```python
from build123d import *

# Parameters (mm, degrees)
F0_W          = 143.1075930595
F0_H          = 104.4075153768
F1_DEPTH      = 12.7
F3_DEPTH      = 25.4
F3_DEPTH_BACK = 25.4
F4_DEPTH      = 25.4
F6_DEPTH      = 25.4


with BuildPart() as f1:
    # F0 (on Top) → F1 (new body)
    with BuildSketch(Plane.XY):
        with Locations((2.4059638381, -20.6538233906)):
            Rectangle(F0_W, F0_H)
    extrude(amount=F1_DEPTH)

    # F2 (on face) → F3 (join, two sides)
    with BuildSketch(Plane.XY.offset(12.7)) as f3_sk:
        with BuildLine():
            Line((15.3577672787, 31.5499342978), (-2.9768298588, 31.5499342978))
            ThreePointArc((-2.9768298588, 31.5499342978), (-24.3292867036, -22.491323871), (4.6469989905, -72.857581079))
            Line((4.6469989905, -72.857581079), (32.5235698655, -72.857581079))
            ThreePointArc((32.5235698655, -72.857581079), (-12.9702679448, -26.7224080826), (15.3577672787, 31.5499342978))
        make_face()
        with BuildLine():
            ThreePointArc((4.6469989905, -72.857581079), (73.6316913936, -76.7914525658), (109.3100037632, -17.6186449826))
            ThreePointArc((109.3100037632, -17.6186449826), (69.2394439219, 43.6714076224), (-2.9768298588, 31.5499342978))
            Line((-2.9768298588, 31.5499342978), (15.3577672787, 31.5499342978))
            ThreePointArc((15.3577672787, 31.5499342978), (42.4015261233, 38.4965408489), (69.4452849679, 31.5499342978))
            Line((69.4452849679, 31.5499342978), (73.9597603679, 31.5499342978))
            Line((73.9597603679, 31.5499342978), (73.9597603679, 28.7816991138))
            ThreePointArc((73.9597603679, 28.7816991138), (91.9989568029, 8.6303350143), (98.5167119547, -17.6186449826))
            ThreePointArc((98.5167119547, -17.6186449826), (91.9989568029, -43.8676249794), (73.9597603679, -64.0189890789))
            Line((73.9597603679, -64.0189890789), (73.9597603679, -72.857581079))
            Line((73.9597603679, -72.857581079), (52.279482381, -72.857581079))
            ThreePointArc((52.279482381, -72.857581079), (42.4015261233, -73.733830814), (32.5235698655, -72.857581079))
            Line((32.5235698655, -72.857581079), (4.6469989905, -72.857581079))
        make_face()
    extrude(amount=F3_DEPTH)
    extrude(f3_sk.sketch, amount=-F3_DEPTH_BACK)

    # F4 (cut): a face of the model
    f4_faces = [f1.faces().sort_by_distance(p)[0] for p in [
        (34.4480932251, -19.6254541978, 12.7),
    ]]
    extrude(f4_faces, amount=-F4_DEPTH, mode=Mode.SUBTRACT)

    # F5 (on Front) → F6 (join)
    with BuildSketch(Plane.XZ):
        Polygon((-24.4303904474, 12.8110842779), (-24.5704315603, 25.2280384302), (-42.8279539842, 12.8110842779), align=None)
    extrude(amount=F6_DEPTH)


solid = f1.part
```
Check sheet for the modelled part. Datum: model origin and axes. Units: mm. A direction names the side the tool comes from. Give positions to 0.01 mm unless a question says otherwise; leave off trailing zeros. Write each loop counter-clockwise with the first axis right and the second up, starting at its lowest first coordinate (ties: lowest second). Pieces come first, ordered by that corner, then holes.
Item 1: Cross-section at B-B (y = 3.5). Enter the section's corners in (x, z).
Item 2: Scan lines: L1, parallel to X at y = -24, z = 23.5 (3 decimals); L2, parallel to Z at x = -57, y = -62; L3, parallel to X at y = 33.5, z = 32. Record each from-to range of solid material in increasing order.
Item 3: Cross-section at A-A (z = 20.5). Enter the section's corners in (x, y).
Item 4: Cross-section at C-C (x = 91). Enter the section's corners in (y, z), and give its area (3 significant figures).
Item 5: Gauge pin test, flat ends, axial feed: pin 1 (2 mm diameter, centred on y = 30, z = 27, fed in from -X); pin 2 (14 mm diameter, centred on x = -31.5, z = 3.5, fed in from +Y); pin 3 (10 mm diameter, centred on x = -31, z = 8, fed in from -Y); pin 4 (5 mm diameter, centred on x = -25.5, y = -17, fed in from +Z). Record the tip position at first contact, or that the pin passes through.
Item 6: Cross-section at D-D (z = 7). Enter the section's corners in (x, y), and give its area (3 significant figures).
Item 7: Access from +Z, -Z, +X, -X, +Y, -Y to the whole of each face (thin tool, end or side, straight path). Record for faces 1 (the face through (-30, -25.4, 16)), 2 (the face through (-37, 31.55, 6)), 3 (the face through (-33, -72.858, 6)), 4 (the face through (-30, 0, 16)), 5 (the face through (7, -62, 38.1)).
Report:
1. outline: (-69.15, 0) - (-21.09, 0) - (-21.09, -12.7) - (-9.59, -12.7) - (-9.59, 38.1) - (-21.09, 38.1) - (-21.09, 12.7) - (-69.15, 12.7) - close; (94.39, -12.7) - (105.89, -12.7) - (105.89, 38.1) - (94.39, 38.1) - close
2. L1: x = -27.111 to -24.551, -24.202 to -13.35, 98.153 to 109.005
2. L2: z = 0 to 12.7
2. L3: x = -0.77 to 19.25, 65.55 to 85.57
3. outline: (-31.52, -25.4) - (-24.52, -25.4) - (-24.52, 0) - (-31.52, 0) - close; circle Ø133.82 at (42.4, -17.62); hole (52.28, -72.86) - (73.96, -72.86) - (73.96, -64.02) arc R56.12 ccw to (73.96, 28.78) - (73.96, 31.55) - (69.45, 31.55) arc R56.12 ccw (long way) to start
4. outline: (-63.61, -12.7) - (-45.67, -12.7) - (-45.67, 38.1) - (-63.61, 38.1) - close; (10.44, -12.7) - (28.37, -12.7) - (28.37, 38.1) - (10.44, 38.1) - close
4. area: 1,820 mm2
5. pin 1: stops at x = -5.59
5. pin 2: stops at y = 31.55
5. pin 3: stops at y = -72.86
5. pin 4: stops at z = 38.1
6. outline: (-69.15, -72.86) - (4.65, -72.86) arc R66.91 ccw (long way) to (-2.98, 31.55) - (-69.15, 31.55) - close; hole (52.28, -72.86) - (73.96, -72.86) - (73.96, -64.02) arc R56.12 ccw to (73.96, 28.78) - (73.96, 31.55) - (69.45, 31.55) arc R56.12 ccw (long way) to start
6. area: 9,560 mm2
7. face 1: +Z, -X, -Y
7. face 2: +Z, -Z, -X, +Y
7. face 3: +Z, -Z, -X, -Y
7. face 4: +Z, -X, +Y
7. face 5: +Z, +X, -X, +Y, -Y
